Source: CAD feature listing. Evaluate the final solid. Frame: model axes, mm. Face numbers are marked on the shaded views. A direction names the side the tool comes from. Round coordinates to 2 decimals unless told otherwise and drop trailing zeros. Loops run counter-clockwise (first coordinate to the right, second up) from the corner with the lowest first, then second, coordinate; pieces in that order, holes last. Notation, with made-up numbers: (-33, 39) - (-19, 39) arc R6 cw to (-19, 50) - close; hole circle Ø1 at (9, 58). An arc over 180 degrees is marked (long way). One line per question, with ' | ' between items. Start each with the question number.
1. Cut plane B-B (z = 12). Return loops of the section in (x, y), then the cut area to 3 significant figures.
2. Cut plane A-A (y = 0). Return loops of the section in (x, z).
3. Ray query, line 1 (Y direction, x = 0, z = 12.25); line 2 (Z direction, x = 0, y = -7.25); line 3 (X direction, y = 2, z = 3.5). Return the intervals inside material, ascending.
4. Cut plane C-C (x = -0.25). State how many separate pieces and enclosed holes the cut face has, then the cut area to 3 significant figures.
5. Cut plane D-D (z = 2.5). Return loops of the section in (x, y).
6. Mould query, pull axis Z, two halves, no side actions, for the marked faces 1, 2 and 3. Classes: pulls with the +Z half, pulls with the -Z half, needs draft (parallel to the pull), parting line crosses it, or undercut.
7. Access query for the marked faces 4 and 5. Directions: +Z, -Z, +X, -X, +Y, -Y. A direction counts if a zero-diameter tool reaches every point of the face in a straight line with its end or side. Return the directions, or none.
8. Pin query (flat end, axial travel): pin 1 (10 mm diameter, centred on y = 4, z = 8.5, fed in from -X); pin 2 (4 mm diameter, centred on y = -7, z = 9.5, fed in from +X); pin 3 (3 mm diameter, centred on x = 0, y = 0, fed in from +Z); pin 4 (2 mm diameter, centred on x = 7.5, z = 10, fed in from +Y). Return the tip coordinate at first contact, or that it passes through.
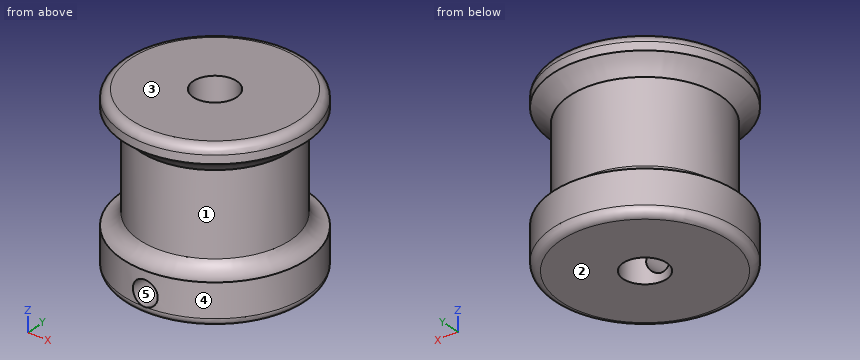
```python
from build123d import *

# Parameters (mm, degrees)
F2_R     = 2.6
F3_DEPTH = 20
F5_R     = 1.5
F6_DEPTH = 10
F7_R     = 1


with BuildPart() as f1:
    # F0 (on Front) → F1 (revolve)
    with BuildSketch(Plane.XZ):
        with BuildLine():
            Line((-11, 0), (0, 0))
            Line((0, 0), (0, 20))
            Line((0, 20), (-11, 20))
            Line((-11, 20), (-11, 18))
            ThreePointArc((-11, 18), (-9.931221, 17.186703), (-9, 16.218938))
            Line((-9, 16.218938), (-9, 6.446878))
            ThreePointArc((-9, 6.446878), (-9.763254, 5.396188), (-11, 5))
            Line((-11, 5), (-11, 0))
        make_face()
    revolve(axis=Axis((0, 0, 10), (0, 0, -1)))

    # F2 (on face) → F3 (cut)
    with BuildSketch(Plane.XY.offset(20)):
        Circle(F2_R)
    extrude(amount=-F3_DEPTH, mode=Mode.SUBTRACT)

    # F5 (on offset) → F6 (cut)
    with BuildSketch(Plane.XZ.offset(11)):
        with Locations((0, 2.5)):
            Circle(F5_R)
    extrude(amount=-F6_DEPTH, mode=Mode.SUBTRACT)

    # F7
    f7_edges = [f1.edges().sort_by_distance(p)[0] for p in [
        (11, 0, 20),
        (11, 0, 0),
    ]]
    fillet(f7_edges, radius=F7_R)


solid = f1.part
```
Answers follow:
1) outline: circle Ø18 at (0, 0); hole circle Ø5.2 at (0, 0) | area: 233 mm2
2) outline: (-11, 1) arc R1 ccw to (-10, 0) - (-2.6, 0) - (-2.6, 20) - (-10, 20) arc R1 ccw to (-11, 19) - (-11, 18) arc R8.72 cw to (-9, 16.22) - (-9, 6.45) arc R2.09 cw to (-11, 5) - close; (2.6, 0) - (10, 0) arc R1 ccw to (11, 1) - (11, 5) arc R2.09 cw to (9, 6.45) - (9, 16.22) arc R8.72 cw to (11, 18) - (11, 19) arc R1 ccw to (10, 20) - (2.6, 20) - close
3) line 1: y = -9 to -2.6, 2.6 to 9 | line 2: z = 0 to 1, 4 to 20 | line 3: x = -10.82 to -1.66, 1.66 to 10.82
4) separate pieces: 3 | enclosed holes: 0 | area: 263 mm2
5) outline: (-1.5, -10.9) - (-1.5, -2.12) arc R2.6 cw (long way) to (1.5, -2.12) - (1.5, -10.9) arc R11 ccw (long way) to start
6) face 1: undercut | face 2: pulls with the -Z half | face 3: pulls with the +Z half
7) face 4: +Z, -Z | face 5: -Y
8) pin 1: stops at x = -10.99 | pin 2: stops at x = 7.48 | pin 3: passes through | pin 4: stops at y = 6.22
